```python
from build123d import *

# Parameters (mm, degrees)
SKETCH1_W           = 100
SKETCH1_H           = 68
BOSS_EXTRUDE1_DEPTH = 6
SKETCH2_W           = 10
SKETCH2_H           = 25
SKETCH2_W_2         = 22
SKETCH2_H_2         = 15
CUT_EXTRUDE1_DEPTH  = 7


with BuildPart() as part:
    # Sketch1 → Boss-Extrude1 (new body)
    with BuildSketch(Plane(origin=(0, 0, 0), x_dir=(1, 0, 0), z_dir=(0, 1, 0))):
        Rectangle(SKETCH1_W, SKETCH1_H)
    extrude(amount=BOSS_EXTRUDE1_DEPTH)

    # Sketch2 → Cut-Extrude1 (cut, through all)
    with BuildSketch(Plane(origin=(0, 6, 0), x_dir=(1, 0, 0), z_dir=(0, 1, 0))):
        with Locations((16.4, -21.5)):
            Rectangle(SKETCH2_W, SKETCH2_H)
        with Locations((-14.6, -26.5)):
            Rectangle(SKETCH2_W_2, SKETCH2_H_2)
    cut_extrude1 = extrude(amount=-CUT_EXTRUDE1_DEPTH, mode=Mode.SUBTRACT)

    # Mirror1: Cut-Extrude1 across plane
    add(cut_extrude1.mirror(Plane.XY), mode=Mode.SUBTRACT)


solid = part.part
```
Work out the finished part from the listing and answer in its coordinate system (mm). A direction names the side the tool comes from. Give positions to 0.01 mm unless a question says otherwise; leave off trailing zeros. Write each loop counter-clockwise with the first axis right and the second up, starting at its lowest first coordinate (ties: lowest second). Pieces come first, ordered by that corner, then holes. Notation, with made-up numbers: (80, 48.25) - (126, 48.25) arc R16 cw to (126, 72.25) - close; hole circle Ø4 at (89, -4.5). An arc over 180 degrees is marked (long way). Use one line per item in the form item = value.
1. Each of these flat-tipped pins is pushed along its axis until it touches: pin 1 Ø1.8 at (x, y) = (14, 3.5) entering from -Z; pin 2 Ø3 at (x, y) = (-15.5, 2.5) entering from +Z; pin 3 Ø3 at (x, y) = (-14, 4.5) entering from -Z. Where does it stop, or does it pass through?
Filled in:
pin_1 = -9
pin_2 = 19
pin_3 = -19
2. Determine the mould class of faces 1 (the face through (21.4, 3, 22)), 2 (the face through (50, 3, 0)), 3 (the face through (-38, 3, -34)), 4 (the face through (-50, 3, 0)) for opening direction X: released by +X, released by -X, zero draft, split by the parting line, or undercut.
Filled in:
face_1 = undercut
face_2 = released by +X
face_3 = zero draft
face_4 = released by -X
3. A cutting plane is placed at C-C (z = -14). Write down the section's boundary in (x, y), and give its area (3 significant figures).
Filled in:
outline = (-50, 0) - (11.4, 0) - (11.4, 6) - (-50, 6) - close; (21.4, 0) - (50, 0) - (50, 6) - (21.4, 6) - close
area = 540 mm^2
4. Consider L1, parallel to X at y = 1.55, z = 28.5; L2, parallel to X at y = 2, z = -13; L3, parallel to Z at x = 13, y = 2. Determine where each line is inside the solid, lowest interval first.
Filled in:
L1 = -50 to -25.6, -3.6 to 11.4, 21.4 to 50
L2 = -50 to 11.4, 21.4 to 50
L3 = -9 to 9
5. For faces 5 (the face through (16, 3, 9)), 6 (the face through (4, 3, 34)), 7 (the face through (16, 3, -9)), determine the directions among +Z, -Z, +X, -X, +Y, -Y from which every point of the face is accessible in a straight line to the end or side of a thin tool.
Filled in:
face_5 = +Z, +Y, -Y
face_6 = +Z, +X, -X, +Y, -Y
face_7 = -Z, +Y, -Y
6. A cutting plane is placed at D-D (x = -17.5). Write down the section's boundary in (y, z), and give its area (3 significant figures).
Filled in:
outline = (0, -19) - (6, -19) - (6, 19) - (0, 19) - close
area = 228 mm^2
7. A cutting plane is placed at B-B (y = 3.65). Write down the section's boundary in (x, z).
Filled in:
outline = (-50, -34) - (-25.6, -34) - (-25.6, -19) - (-3.6, -19) - (-3.6, -34) - (11.4, -34) - (11.4, -9) - (21.4, -9) - (21.4, -34) - (50, -34) - (50, 34) - (21.4, 34) - (21.4, 9) - (11.4, 9) - (11.4, 34) - (-3.6, 34) - (-3.6, 19) - (-25.6, 19) - (-25.6, 34) - (-50, 34) - close
8. A cutting plane is placed at A-A (z = 25). Write down the section's boundary in (x, y), and give its area (3 significant figures).
Filled in:
outline = (-50, 0) - (-25.6, 0) - (-25.6, 6) - (-50, 6) - close; (-3.6, 0) - (11.4, 0) - (11.4, 6) - (-3.6, 6) - close; (21.4, 0) - (50, 0) - (50, 6) - (21.4, 6) - close
area = 408 mm^2
